Can you work these out from the model? Positions are in its coordinate system, mm. A direction names the side the tool comes from. Round coordinates to 2 decimals unless told otherwise and drop trailing zeros. Order: outer loops, then holes, each group sorted by start corner. A loop starts at its lowest first (then second) coordinate and runs counter-clockwise, first axis right, second up. Notation, with made-up numbers: M -25.75,59 L 27.25,59 A8 ccw 27.25,67 Z; hole C -16.75,55 d5. An arc over 180 degrees is marked long. One line per question, with ' | ' between items.
```python
from build123d import *


with BuildPart() as f1:
    # F0 (on Front) → F1 (revolve)
    with BuildSketch(Plane.XZ):
        with BuildLine():
            Line((-6.35, -4.550833), (-6.35, 20.849167))
            Line((-6.35, 20.849167), (-24.638, 20.849167))
            ThreePointArc((-24.638, 20.849167), (-25.176815, 20.625982), (-25.4, 20.087167))
            Line((-25.4, 20.087167), (-25.4, 18.699073))
            ThreePointArc((-25.4, 18.699073), (-25.145088, 17.840068), (-24.462878, 17.259156))
            Line((-24.462878, 17.259156), (-18.399359, 14.573883))
            ThreePointArc((-18.399359, 14.573883), (-17.023935, 13.402689), (-16.51, 11.670824))
            Line((-16.51, 11.670824), (-16.51, 10.778493))
            ThreePointArc((-16.51, 10.778493), (-17.04503, 9.014638), (-18.469799, 7.84525))
            Line((-18.469799, 7.84525), (-24.427939, 5.376878))
            ThreePointArc((-24.427939, 5.376878), (-25.134625, 4.796861), (-25.4, 3.921989))
            Line((-25.4, 3.921989), (-25.4, 2.561167))
            ThreePointArc((-25.4, 2.561167), (-25.176815, 2.022352), (-24.638, 1.799167))
            Line((-24.638, 1.799167), (-15.875, 1.799167))
            Line((-15.875, 1.799167), (-15.875, -4.550833))
            Line((-15.875, -4.550833), (-6.35, -4.550833))
        make_face()
    revolve(axis=Axis((0, 0, 0.052916), (0, 0, 1)))


solid = f1.part
```
(1) On a 3-axis mill with a long thin cutter (end or side, diameter ignored), from which of +Z, -Z, +X, -X, +Y, -Y can I reach the whole of each face in a straight line? I mean faces 4 (the conical face through (4.052, 18.249, 14.704)), 5 (the flat face through (0.3, 16.1, 1.799)), 6 (the cylindrical face through (1.38, 6.2, 8.33)). Say none if no direction works.
Final values:
face 4: none | face 5: -Z | face 6: +Z, -Z
(2) Please list where these lines run through material, in increasing order: probe 1 along Y at (x, z) = (0, 11); probe 2 along Y at (x, z) = (0, -1.75) (3 decimals). Write a range as [from, to].
Final values:
probe 1: [-16.51, -6.35], [6.35, 16.51] | probe 2: [-15.875, -6.35], [6.35, 15.875]
(3) Will these pins go through, and if not, where does the flat tip stop? pin 1 Ø11.5 at (x, y) = (0, 0) entering from -Z; pin 2 Ø8 at (y, z) = (2.5, 10.5) entering from -X; pin 3 Ø12 at (x, z) = (-10, 6.5) entering from -Y; pin 4 Ø6 at (y, z) = (-14, 8) entering from +X.
Final values:
pin 1: through | pin 2: x = -21.58 | pin 3: y = -24.99 | pin 4: x = 21.1
(4) If we section it at C-C on z = 9.75: Please give me the cut outline in (x, y).
Final values:
outline: C 0,0 d33.36; hole C 0,0 d12.7
(5) Thinking about a two-plate mould opening in Z: for faces 1 (the cylindrical face through (-15.748, -4.959, 11.218)), 2 (the cylindrical face through (5.506, 24.796, 19.383)), 3 (the flat face through (5, 5, 20.849)), which applies, released by +Z, released by -Z, zero draft, split by the parting line, or undercut?
Final values:
face 1: undercut | face 2: zero draft | face 3: released by +Z
(6) If we section it at D-D on z = 6.25: Please give me the cut outline in (x, y), plus the area to 3 significant figures.
Final values:
outline: C 0,0 d44.64; hole C 0,0 d12.7 | area: 1,440 mm^2
